Geometry: final body of the model. Coordinates: model frame, mm. Face numbers are marked on the shaded views. A direction names the side the tool comes from. Give positions to 0.01 mm unless a question says otherwise; leave off trailing zeros. Loops run counter-clockwise (first coordinate to the right, second up) from the corner with the lowest first, then second, coordinate; pieces in that order, holes last. Notation, with made-up numbers: (-32, 81) -> (-27, 81) arc R14 cw to (-27, 100) -> close; hole circle Ø5 at (64.5, 21.25). An arc over 180 degrees is marked (long way). Answer in a Markdown table with one row per item. Add a question column.
1) Access query for the marked faces 1, 2 and 3. Directions: +Z, -Z, +X, -X, +Y, -Y. A direction counts if a zero-diameter tool reaches every point of the face in a straight line with its end or side. Return the directions, or none.
2) First-contact query: P1, Ø2, axis at x = 4, z = -9, coming from the -Y side; P2, Ø12, axis at y = 26, z = 6, coming from the +X side; P3, Ø2, axis at x = 9, z = 1, coming from the -Y side. Flat tips, straight axial feed; report the tip coordinate or a pass-through.
3) Line query: line 1 (X direction, y = 10, z = 0); line 2 (X direction, y = 26, z = 12); line 3 (Y direction, x = 1.5, z = -7). Output: solid intervals per line, ascending. Write a range as from..to.
4) Section query A-A (y = 10). Return the cut outline in (x, z), plus the area to 3 significant figures.
```python
from build123d import *

# Parameters (mm, degrees)
SKETCH2_R          = 1.5
CUT_EXTRUDE1_DEPTH = 1


with BuildPart() as part:
    # Sketch1 → Revolve1 (revolve)
    with BuildSketch(Plane.XY, mode=Mode.PRIVATE) as revolve1_sk:
        with BuildLine():
            Line((20, 0), (20, 29.13905258))
            ThreePointArc((20, 29.13905258), (15.995992564, 38.368383693), (9, 45.598094362))
            Line((9, 45.598094362), (9, 50))
            Line((9, 50), (0, 50))
            Line((0, 50), (0, 43.972671684))
            Line((0, 43.972671684), (7.83466695, 43.972671684))
            ThreePointArc((7.83466695, 43.972671684), (14.270082218, 37.351024326), (18, 28.904220391))
            Line((18, 28.904220391), (18, 0))
            Line((18, 0), (20, 0))
        make_face()
    revolve(revolve1_sk.sketch.rotate(Axis((0, 0, 0), (0, 1, 0)), 90), axis=Axis((0, 0, 0), (0, 1, 0)))

    # Sketch2 → Cut-Extrude1 (cut)
    with BuildSketch(Plane.XY.offset(20)):
        with Locations((0, 17.347366398)):
            Circle(SKETCH2_R)
    extrude(amount=-CUT_EXTRUDE1_DEPTH, mode=Mode.SUBTRACT)


solid = part.part
```
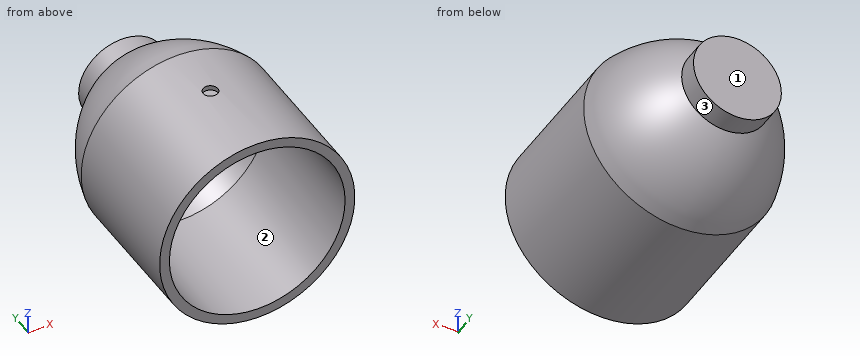
Evaluation:
| question | item | result |
|---|---|---|
| 1 | face 1 | +Z, -Z, +X, -X, +Y |
| 1 | face 2 | -Y |
| 1 | face 3 | +Y |
| 2 | P1 | y = 41.45 |
| 2 | P2 | x = 20 |
| 2 | P3 | y = 42.19 |
| 3 | line 1 | -20..-18, 18..20 |
| 3 | line 2 | -16..-13.42, 13.42..16 |
| 3 | line 3 | 43.97..50 |
| 4 | outline | circle Ø40 at (0, 0); hole circle Ø36 at (0, 0) |
| 4 | area | 239 mm² |
